Autodesk Fusion 360 part; units mm, degrees
sketch "Sketch1" plane through (0, 0, 0) normal (0, 0, 1) x (1, 0, 0)
  line L0 (5, 7.5) -> (-5, 7.5)
  line L1 (-5, 7.5) -> (-5, -7.5)
  line L2 (-5, -7.5) -> (5, -7.5)
  line L3 (5, -7.5) -> (5, 7.5)
  line L4 (5, 7.5) -> (-5, -7.5) construction
  line L5 (-5, 7.5) -> (5, -7.5) construction
  line L6 (-5, 7.5) -> (5, 7.5)
  line L7 (5, 7.5) -> (5, 3)
  line L8 (5, 3) -> (-5, 3)
  line L9 (-5, 3) -> (-5, 7.5)
  line L10 (-5, -7.5) -> (5, -7.5)
  line L11 (5, -7.5) -> (5, -3)
  line L12 (5, -3) -> (-5, -3)
  line L13 (-5, -3) -> (-5, -7.5)
  dimension "d1" = 10
  dimension "d2" = 15
  dimension "d3" = 4.5
  dimension "d4" = 4.5
extrude "Extrude1" add sketch "Sketch1" along normal blind 3 makes body 1
extrude "Extrude2" add sketch "Sketch1" along normal blind 8 contours L0 L1 L3 L6 L7 L8 L9 | L1 L2 L3 L10 L11 L12 L13 bodies 1
fillet "Fillet1" radius 2 2 edges at (0, -3, 3) (0, 3, 3) on bodies 1
fillet "Fillet2" radius 2.5 2 edges at (0, -7.5, 0) (0, 7.5, 0) on bodies 1
sketch "Sketch2" plane through (0, 0, 0) normal (0, 0, 1) x (1, 0, 0)
  circle A0 centre (20, 0) radius 4
  circle A1 centre (20, 0) radius 9
  dimension "d13" = 8
  dimension "d14" = 18
extrude "Extrude3" add sketch "Sketch2" along normal blind 20 separate body makes body 2
delete_body "RemoveBody1" bodies 2
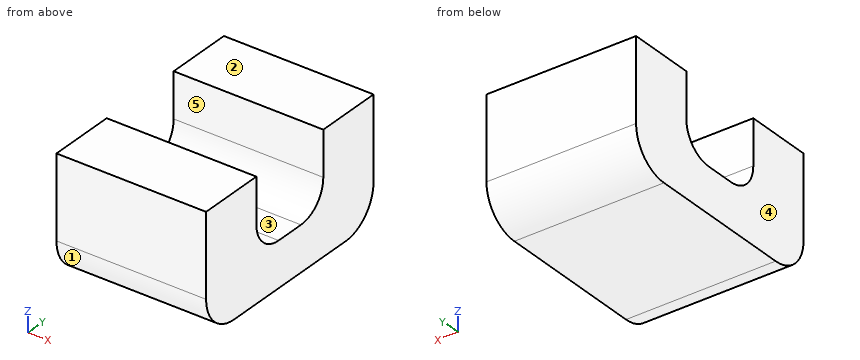
Check sheet for the modelled part. Datum: model origin and axes. Units: mm. Face numbers are marked on the shaded views. A direction names the side the tool comes from. Coordinates: 2 decimals unless noted, no trailing zeros. Loops run counter-clockwise (first coordinate to the right, second up) from the corner with the lowest first, then second, coordinate; pieces in that order, holes last. Notation, with made-up numbers: M 89.25,27 L 125.25,27 A12 cw 125.25,36 Z; hole C 82.5,85 d5. An arc over 180 degrees is marked long. Answer as a JSON object with one key per item and string values.
1. Release check for a two-part mould opening along Y. For the marked faces 1, 2 and 3 record: pulls with the +Y half, pulls with the -Y half, needs draft (parallel to the pull), parting line crosses it, or undercut.
Outcome:
{"face 1": "pulls with the -Y half", "face 2": "needs draft", "face 3": "undercut"}
2. Sectioned sample at A-A on z = 7.75. Record the cut outline in (x, y), and give its area (3 significant figures).
Outcome:
{"outline": "M -5,-7.5 L 5,-7.5 L 5,-3 L -5,-3 Z; M -5,3 L 5,3 L 5,7.5 L -5,7.5 Z", "area": "90.0 mm²"}
3. Depth check by flat-ended pin: P1, Ø1, axis at x = 0.5, y = -0.5, coming from the +Z side; P2, Ø4, axis at x = -3, y = 0.5, coming from the +Z side. Enter the tip coordinate at first touch or a pass-through.
Outcome:
{"P1": "z = 3", "P2": "z = 3.68"}
4. Sectioned sample at B-B on x = 1. Record the cut outline in (y, z), and give its area (3 significant figures).
Outcome:
{"outline": "M -7.5,2.5 A2.5 ccw -5,0 L 5,0 A2.5 ccw 7.5,2.5 L 7.5,8 L 3,8 L 3,5 A2 cw 1,3 L -1,3 A2 cw -3,5 L -3,8 L -7.5,8 Z", "area": "89.0 mm²"}
5. Scan lines: L1, parallel to Y at x = 1, z = 7; L2, parallel to Z at x = 2.5, y = -0.75; L3, parallel to Y at x = -3.5, z = 3.5. Record each from-to range of solid material in increasing order. Write a range as from..to.
Outcome:
{"L1": "-7.5..-3, 3..7.5", "L2": "0..3", "L3": "-7.5..-2.32, 2.32..7.5"}
6. Sectioned sample at C-C on z = 1. Record the cut outline in (x, y), and give its area (3 significant figures).
Outcome:
{"outline": "M -5,-7 L 5,-7 L 5,7 L -5,7 Z", "area": "140 mm²"}
7. Sectioned sample at D-D on y = 0. Record the cut outline in (x, z), and give its area (3 significant figures).
Outcome:
{"outline": "M -5,0 L 5,0 L 5,3 L -5,3 Z", "area": "30.0 mm²"}
8. Access from +Z, -Z, +X, -X, +Y, -Y to the whole of each face (thin tool, end or side, straight path). Record for the marked faces 4 and 5.
Outcome:
{"face 4": "+Z, -Z, -X, +Y, -Y", "face 5": "+Z, +X, -X"}
